Read the model definition and answer for the solid it produces. Units are mm, in the model's axes. A direction names the side the tool comes from. Coordinates: 2 decimals unless noted, no trailing zeros. Write each loop counter-clockwise with the first axis right and the second up, starting at its lowest first coordinate (ties: lowest second). Pieces come first, ordered by that corner, then holes.
from build123d import *

# Parameters (mm, degrees)
F0_W     = 70
F0_H     = 12.5
F0_R     = 2
F0_R_2   = 1.5
F0_R_3   = 4.1
F0_W_2   = 2
F1_DEPTH = 3
F2_R     = 0.5
F3_R     = 2.625
F3_R_2   = 1.5
F4_DEPTH = 1.5
F5_R     = 1


with BuildPart() as f1:
    # F0 (on Top) → F1 (new body)
    with BuildSketch(Plane.XY):
        Rectangle(F0_W, F0_H)
        with Locations((-30.725, 0)):
            Circle(F0_R, mode=Mode.SUBTRACT)
        with Locations((-23.762, 0)):
            Circle(F0_R_2, mode=Mode.SUBTRACT)
        with Locations((-13.05, 0)):
            Circle(F0_R_3, mode=Mode.SUBTRACT)
        Circle(F0_R_2, mode=Mode.SUBTRACT)
        with Locations((13.05, 0)):
            Circle(F0_R_3, mode=Mode.SUBTRACT)
        with Locations((23.762, 0)):
            Circle(F0_R_2, mode=Mode.SUBTRACT)
        with Locations((30.725, 0)):
            Circle(F0_R, mode=Mode.SUBTRACT)
        with Locations((36, 0)):
            Rectangle(F0_W_2, F0_H)
        with Locations((-36, 0)):
            Rectangle(F0_W_2, F0_H)
    extrude(amount=F1_DEPTH)

    # F2
    f2_edges = [f1.edges().sort_by_distance(p)[0] for p in [
        (-17.15, 0, 3),
        (8.95, 0, 3),
    ]]
    fillet(f2_edges, radius=F2_R)

    # F3 (on face) → F4 (cut)
    with BuildSketch(Plane.XY.offset(3)):
        with Locations((-23.762, 0)):
            Circle(F3_R)
        with Locations((-23.762, 0)):
            Circle(F3_R_2, mode=Mode.SUBTRACT)
        Circle(F3_R)
        Circle(F3_R_2, mode=Mode.SUBTRACT)
        with Locations((23.762, 0)):
            Circle(F3_R)
        with Locations((23.762, 0)):
            Circle(F3_R_2, mode=Mode.SUBTRACT)
    extrude(amount=-F4_DEPTH, mode=Mode.SUBTRACT)

    # F5
    f5_edges = [f1.edges().sort_by_distance(p)[0] for p in [
        (0, 6.25, 3),
        (-37, 0, 3),
        (0, -6.25, 3),
        (37, 0, 3),
        (-37, 6.25, 1.5),
        (-37, -6.25, 1.5),
        (37, 6.25, 1.5),
        (37, -6.25, 1.5),
    ]]
    fillet(f5_edges, radius=F5_R)


solid = f1.part
Item 1: Given pin 1 (2.5 mm diameter, centred on x = -1, y = 0, fed in from +Z), flat-ended and moving along its own axis, determine where the tip first touches the part or whether it passes through.
Item 2: The part is cut by section D-D (x = 0). Give the vertices of the cut face in (y, z) (3 decimals).
Item 3: Find the intervals of material crossed by probe 1 along X at (y, z) = (3.5, 0.25); probe 2 along X at (y, z) = (1.75, 1.45); probe 3 along Y at (x, z) = (-15, 1.7), in increasing order.
Item 4: The part is cut by section B-B (z = 0.5). Give the vertices of the cut face in (x, y) (3 decimals).
Item 5: The part is cut by section C-C (y = 0). State how many separate pieces and enclosed holes the cut face has, and give its area (3 significant figures).
Item 6: For faces 4 (the cylindrical face through (-32.723, 0.088, 1.479)), 5 (the cylindrical face through (-21.34, -1.01, 2.26)), determine the directions among +Z, -Z, +X, -X, +Y, -Y from which every point of the face is accessible in a straight line to the end or side of a thin tool.
Item 7: The part is cut by section A-A (x = 13.05). Give the vertices of the cut face in (y, z).
Item 8: Determine the mould class of faces 1 (the flat face through (-1, -6.25, 1)), 2 (the flat face through (-1, 3, 0)), 3 (the cylindrical face through (22.263, 0.066, 0.74)) for opening direction Y: +Y half, -Y half, draft (parallel to the pull), parting line (faces both ways), or undercut.
Answer:
1. pin 1: stops at z = 1.5
2. outline: (-6.25, 0) - (-1.5, 0) - (-1.5, 1.5) - (-2.625, 1.5) - (-2.625, 3) - (-5.25, 3) arc R1 ccw to (-6.25, 2) - close; (1.5, 0) - (6.25, 0) - (6.25, 2) arc R1 ccw to (5.25, 3) - (2.625, 3) - (2.625, 1.5) - (1.5, 1.5) - close
3. probe 1: x = -37 to -15.19, -10.91 to 10.91, 15.19 to 37
3. probe 2: x = -37 to -31.69, -29.76 to -16.76, -9.34 to 9.34, 16.76 to 29.76, 31.69 to 37
3. probe 3: y = -6.25 to -3.61, 3.61 to 6.25
4. outline: (-37, -5.25) arc R1 ccw to (-36, -6.25) - (36, -6.25) arc R1 ccw to (37, -5.25) - (37, 5.25) arc R1 ccw to (36, 6.25) - (-36, 6.25) arc R1 ccw to (-37, 5.25) - close; hole circle Ø4 at (-30.725, 0); hole circle Ø3 at (-23.762, 0); hole circle Ø8.2 at (-13.05, 0); hole circle Ø3 at (0, 0); hole circle Ø8.2 at (13.05, 0); hole circle Ø3 at (23.762, 0); hole circle Ø4 at (30.725, 0)
5. separate pieces: 8
5. enclosed holes: 0
5. area: 111 mm2
6. face 4: +Z, -Z
6. face 5: +Z
7. outline: (-6.25, 0) - (-4.1, 0) - (-4.1, 2.5) arc R0.5 ccw to (-4.6, 3) - (-5.25, 3) arc R1 ccw to (-6.25, 2) - close; (4.1, 0) - (6.25, 0) - (6.25, 2) arc R1 ccw to (5.25, 3) - (4.6, 3) arc R0.5 ccw to (4.1, 2.5) - close
8. face 1: -Y half
8. face 2: draft
8. face 3: undercut
